Answer from the drawing. Dimensions are ordinates in mm from the lowest x, y and z of the part. A direction names the side the tool comes from. Coordinates: 2 decimals unless noted, no trailing zeros. Write each loop counter-clockwise with the first axis right and the second up, starting at its lowest first coordinate (ties: lowest second). Pieces come first, ordered by that corner, then holes. Notation, with made-up numbers: (39.25, 56.5) -> (87.25, 56.5) arc R12 cw to (87.25, 61.5) -> close; hole circle Ø7 at (-6.5, 57.5). An arc over 180 degrees is marked (long way). One line per item, written item: value. Start each with the question number.
1. Find section A-A, the plane z = 23.25. Write down the section's boundary in (x, y) (1 decimal).
2. For the marked faces 4 and 5, determine the directions among +Z, -Z, +X, -X, +Y, -Y from which every point of the face is accessible in a straight line to the end or side of a thin tool.
3. Given P1, Ø12, axis at x = 70.5, z = 23, coming from the +Y side; P2, Ø18, axis at x = 15, y = 156.03, coming from the +Z side; P3, Ø2, axis at y = 83, z = 23, coming from the -X side; P4, Ø8, axis at x = 50.5, z = 16, coming from the -Y side (1 decimal), each flat-ended and moving along its own axis, determine where each tip first touches the part or whether it passes through.
4. Consider line 1 along Y through (x, z) = (15, 23.75); line 2 along X through (y, z) = (156.5, 24.5); line 3 along Z through (x, y) = (47, 57). Determine where each line is inside the solid, lowest interval first.
5. Find section C-C, the plane x = 19. Write down the section's boundary in (y, z) (1 decimal).
6. Find section B-B, the plane y = 159. Write down the section's boundary in (x, z).
7. Find section D-D, the plane y = 36. Write down the section's boundary in (x, z).
8. For a pull along Y with two mould halves and no side action, classify the marked faces 1, 2 and 3 as pulls with the +Y half, pulls with the -Y half, needs draft (parallel to the pull), parting line crosses it, or undercut.
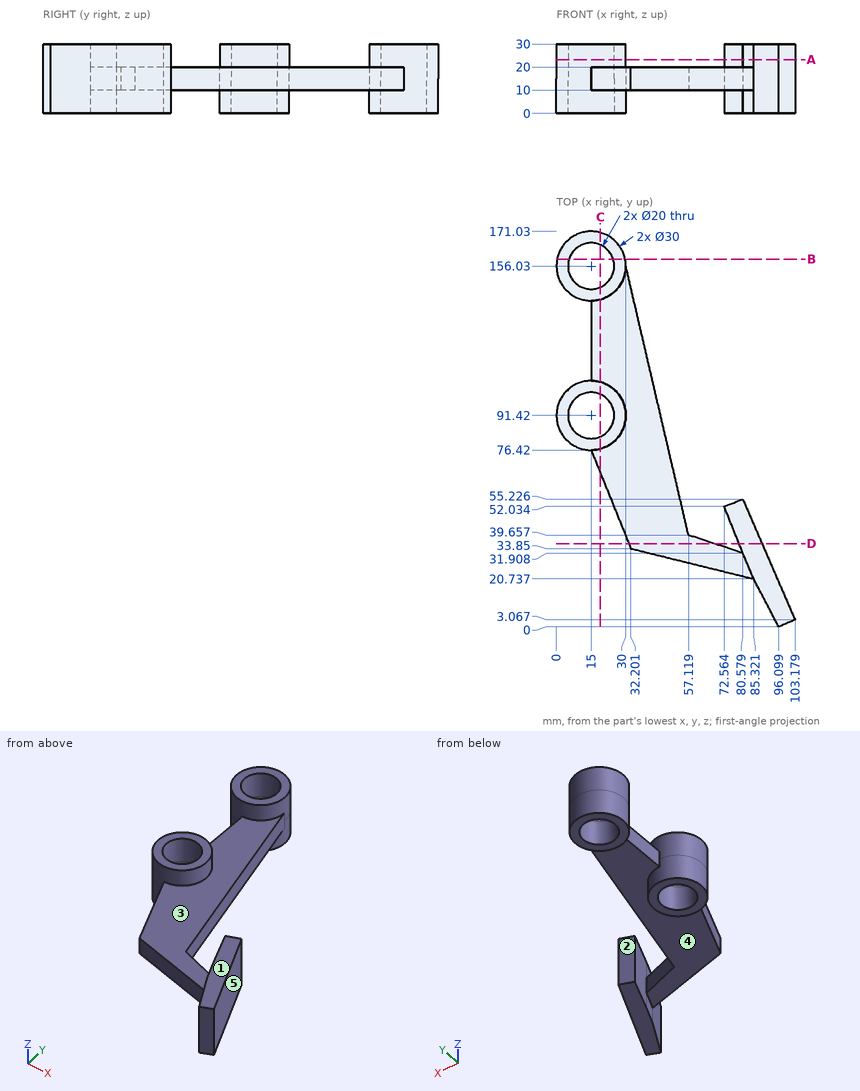
Answer block:
1. outline: circle Ø30 at (15, 91.4); circle Ø30 at (15, 156); (72.6, 52) -> (80.6, 31.9) -> (85.3, 20.7) -> (96.1, 0) -> (103.2, 3.1) -> (80.6, 55.2) -> close; hole circle Ø20 at (15, 91.4); hole circle Ø20 at (15, 156)
2. face 4: -Z
2. face 5: +Z, -Z, +X, +Y
3. P1: stops at y = 53.6
3. P2: passes through
3. P3: stops at x = 1.96
3. P4: stops at y = 28.3
4. line 1: y = 76.42 to 81.42, 101.42 to 106.42, 141.03 to 146.03, 166.03 to 171.03
4. line 2: x = 0.01 to 5.01, 24.99 to 29.99
4. line 3: z = 10 to 20
5. outline: (66.5, 10) -> (77, 10) -> (77, 0) -> (82.3, 0) -> (82.3, 30) -> (77, 30) -> (77, 20) -> (66.5, 20) -> close; (100.6, 0) -> (105.9, 0) -> (105.9, 10) -> (141.6, 10) -> (141.6, 0) -> (146.9, 0) -> (146.9, 30) -> (141.6, 30) -> (141.6, 20) -> (105.9, 20) -> (105.9, 30) -> (100.6, 30) -> close; (165.2, 0) -> (170.5, 0) -> (170.5, 30) -> (165.2, 30) -> close
6. outline: (0.3, 0) -> (5.45, 0) -> (5.45, 30) -> (0.3, 30) -> close; (24.55, 0) -> (29.7, 0) -> (29.7, 30) -> (24.55, 30) -> close
7. outline: (31.33, 10) -> (68.19, 10) -> (68.19, 20) -> (31.33, 20) -> close; (78.95, 0) -> (88.91, 0) -> (88.91, 30) -> (78.95, 30) -> close
8. face 1: needs draft
8. face 2: pulls with the +Y half
8. face 3: undercut
